Design review of the part built by this model. Coordinates are the model's own, in mm. Face numbers are marked on the shaded views. A direction names the side the tool comes from. Give positions to 0.01 mm unless a question says otherwise; leave off trailing zeros. Loops run counter-clockwise (first coordinate to the right, second up) from the corner with the lowest first, then second, coordinate; pieces in that order, holes last. Notation, with made-up numbers: (36.25, 88) -> (58.25, 88) arc R8 cw to (58.25, 93) -> close; hole circle Ø5 at (79.25, 68.25). An arc over 180 degrees is marked (long way). Use CSV: the item, a comma, the result in double quotes. Start each with the question number.
Item 1: We need section B-B (x = 22.5). State the section outline as (y, z) points.
Item 2: We need section C-C (y = 5.5). State the section outline as (x, z) points.
Item 3: For the marked faces 1, 2 and 3, list the 3-axis set-ups (+Z, -Z, +X, -X, +Y, -Y) from which the entire face can be reached by the end or side of a thin tool; tool diameter is ignored.
Item 4: We need section A-A (z = 5.75). State the section outline as (x, y) points, plus the area to 3 significant figures.
Item 5: We need section D-D (x = 41). State the section outline as (y, z) points.
Item 6: Wall thickness on line 1 along Y through (x, z) = (36, 3.5); line 2 along X through (y, z) = (3.5, 6.5): over which ranges is each line inside the solid? List them lowest first. Write a range as from..to.
Item 7: Clearance check with flat-ended pins moving along their axes: pin 1 (3 mm diameter, centred on x = 19, z = 3, fed in from +Y); pin 2 (1 mm diameter, centred on y = -1.5, z = 8, fed in from +X); pin 3 (5 mm diameter, centred on y = 12.5, z = 6.5, fed in from -X). State where each tip first meets the part, or that it passes through.
from build123d import *

# Parameters (mm, degrees)
SKETCH2_W           = 45
SKETCH2_H           = 20
BOSS_EXTRUDE1_DEPTH = 1
SKETCH3_R           = 12.5
BOSS_EXTRUDE4_DEPTH = 8
SKETCH6_W           = 10
SKETCH6_H           = 1
BOSS_EXTRUDE5_DEPTH = 7


with BuildPart() as part:
    # Sketch2 → Boss-Extrude1 (new body)
    with BuildSketch(Plane.XY):
        with Locations((22.5, 10)):
            Rectangle(SKETCH2_W, SKETCH2_H)
    extrude(amount=BOSS_EXTRUDE1_DEPTH)

    # Sketch3 → Boss-Extrude4 (add)
    with BuildSketch(Plane.XY.offset(1)):
        with Locations(Location((22.5, 5.5, 0), (0, 0, 206.103881137))):
            Circle(SKETCH3_R)
    extrude(amount=BOSS_EXTRUDE4_DEPTH)

    # Sketch6 → Boss-Extrude5 (add)
    with BuildSketch(Plane.XY.offset(1)):
        with Locations((5, 0.5)):
            Rectangle(SKETCH6_W, SKETCH6_H)
        with Locations((40, 0.5)):
            Rectangle(SKETCH6_W, SKETCH6_H)
    extrude(amount=BOSS_EXTRUDE5_DEPTH)


solid = part.part
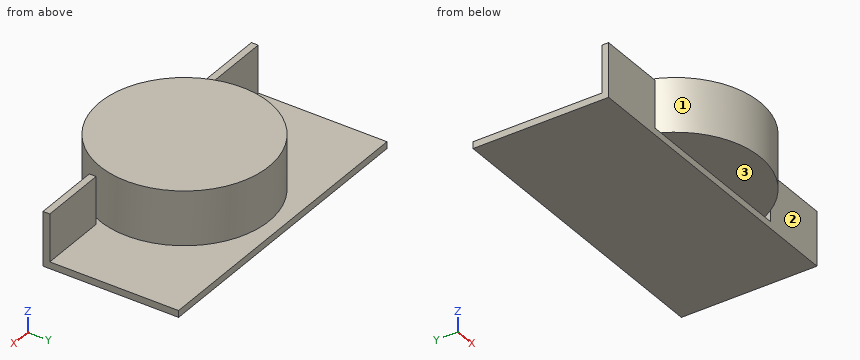
Results found:
1,outline,"(-7, 1) -> (0, 1) -> (0, 0) -> (20, 0) -> (20, 1) -> (18, 1) -> (18, 9) -> (-7, 9) -> close"
2,outline,"(0, 0) -> (45, 0) -> (45, 1) -> (35, 1) -> (35, 9) -> (10, 9) -> (10, 1) -> (0, 1) -> close"
3,face 1,"+Z"
3,face 2,"-Z, -Y"
3,face 3,"-Z, +X, -X, -Y"
4,outline,"(0, 0) -> (10, 0) -> (10, 1) -> (0, 1) -> close; circle Ø25 at (22.5, 5.5); (35, 0) -> (45, 0) -> (45, 1) -> (35, 1) -> close"
4,area,"511 mm²"
5,outline,"(0, 0) -> (20, 0) -> (20, 1) -> (1, 1) -> (1, 8) -> (0, 8) -> close"
6,line 1,"0..1"
6,line 2,"10.16..34.84"
7,pin 1,"y = 17.84"
7,pin 2,"x = 33.18"
7,pin 3,"x = 10.84"
